from build123d import *

# Parameters (mm, degrees)
SKETCH2_R           = 12.5
BOSS_EXTRUDE1_DEPTH = 30
SKETCH3_W           = 30
SKETCH3_H           = 30
BOSS_EXTRUDE2_DEPTH = 40
SKETCH4_W           = 10
SKETCH4_H           = 20
CUT_EXTRUDE1_DEPTH  = 40
FILLET1_R           = 15
SKETCH5_R           = 5
CUT_EXTRUDE2_DEPTH  = 40


with BuildPart() as part:
    # Sketch2 → Boss-Extrude1 (new body)
    with BuildSketch(Plane.XY):
        Circle(SKETCH2_R)
    extrude(amount=BOSS_EXTRUDE1_DEPTH)

    # Sketch3 → Boss-Extrude2 (add)
    with BuildSketch(Plane.XY.offset(30)):
        Rectangle(SKETCH3_W, SKETCH3_H)
    extrude(amount=BOSS_EXTRUDE2_DEPTH)

    # Sketch4 → Cut-Extrude1 (cut)
    with BuildSketch(Plane(origin=(0, 15, 0), x_dir=(1, 0, 0), z_dir=(0, 1, 0))):
        with Locations((0, -60)):
            Rectangle(SKETCH4_W, SKETCH4_H)
    extrude(amount=-CUT_EXTRUDE1_DEPTH, mode=Mode.SUBTRACT)

    # Fillet1
    fillet1_edges = [part.edges().sort_by_distance(p)[0] for p in [
        (10, 15, 70),
        (10, -15, 70),
        (-10, -15, 70),
        (-10, 15, 70),
    ]]
    fillet(fillet1_edges, radius=FILLET1_R - 0.0001)  # a hair under: the kernel refuses the full size

    # Sketch5 → Cut-Extrude2 (cut)
    with BuildSketch(Plane.ZY.offset(15)):
        with Locations(Location((55, 0, 0), (0, 0, 270))):
            Circle(SKETCH5_R)
    extrude(amount=-CUT_EXTRUDE2_DEPTH, mode=Mode.SUBTRACT)


solid = part.part
The model under review builds one solid part; all positions refer to its coordinate system, in mm. A direction names the side the tool comes from. Round coordinates to 2 decimals unless told otherwise and drop trailing zeros. Loops run counter-clockwise (first coordinate to the right, second up) from the corner with the lowest first, then second, coordinate; pieces in that order, holes last. Notation, with made-up numbers: M 58.5,42.5 L 117.5,42.5 A21 ccw 117.5,78.5 Z; hole C 44.25,23 d7. An arc over 180 degrees is marked long. Answer as CSV lines item,"result". Start each with the question number.
Item 1: Consider section B-B (y = 4). Write out the cut boundary in (x, z).
Item 2: For faces 4 (the face through (10.07, -10.72, 65.49)), 5 (the face through (-5, 0, 62)), 6 (the face through (-14, 0, 30)), list the 3-axis set-ups (+Z, -Z, +X, -X, +Y, -Y) from which the entire face can be reached by the end or side of a thin tool; tool diameter is ignored.
Item 3: Consider section D-D (z = 27). Write out the cut boundary in (x, y).
Item 4: Wall thickness on line 1 (Y direction, x = -10.25, z = 55); line 2 (Z direction, x = -8, y = 0): over which ranges is each line inside the solid? List them lowest first. Write a range as [from, to].
Item 5: Mouldability with a two-part tool opening along X and no side actions: class faces 1 (the face through (-15, -0.2, 49.7)), 2 (the face through (15, -0.2, 49.7)), 3 (the face through (0, 0, 50)) as released by +X, released by -X, zero draft, split by the parting line, or undercut.
Item 6: Consider section C-C (x = 0). Write out the cut boundary in (y, z), then the cut area to 3 significant figures.
Item 7: Insertion check: P1, Ø3, axis at x = -5, y = 5, coming from the -Z side; P2, Ø8, axis at x = 9.5, z = 61.5, coming from the +Y side; P3, Ø6, axis at x = 6, y = 7.5, coming from the +Z side; P4, Ø8, axis at x = 11.5, y = -9.5, coming from the +Z side. Each pin has a flat end and moves straight along its axis. Give the tip position at first contact, or say it passes through.
Answer:
1,outline,"M -15,30 L -11.84,30 L -11.84,0 L 11.84,0 L 11.84,30 L 15,30 L 15,52 L 5,52 L 5,50 L -5,50 L -5,52 L -15,52 Z; M -15,58 L -5,58 L -5,69.46 L -15,69.46 Z; M 5,58 L 15,58 L 15,69.46 L 5,69.46 Z"
2,face 4,"+Z, +X, -X, -Y"
2,face 5,"+Z, +Y, -Y"
2,face 6,"-Z"
3,outline,"C 0,0 d25"
4,line 1,"y = [-15, -5], [5, 15]"
4,line 2,"z = [0, 50], [60, 70]"
5,face 1,"released by -X"
5,face 2,"released by +X"
5,face 3,"undercut"
6,outline,"M -15,30 L -12.5,30 L -12.5,0 L 12.5,0 L 12.5,30 L 15,30 L 15,50 L -15,50 Z"
6,area,"1,350 mm^2"
7,P1,"stops at z = 0"
7,P2,"stops at y = 14.79"
7,P3,"stops at z = 69.31"
7,P4,"stops at z = 68.96"
